Design review of the part built by this model. Coordinates are the model's own, in mm. A direction names the side the tool comes from. Coordinates: 2 decimals unless noted, no trailing zeros. Loops run counter-clockwise (first coordinate to the right, second up) from the corner with the lowest first, then second, coordinate; pieces in that order, holes last. Notation, with made-up numbers: M 11.5,82.5 L 67.5,82.5 A11 cw 67.5,92.5 Z; hole C 4.5,-39.5 d3. An arc over 180 degrees is marked long. Answer as a JSON object with one key per item and string values. Group by question number.
1. Consider section A-A (x = 0). State the section outline as (y, z) points.
2. Insertion check: pin 1 (6 mm diameter, centred on y = 3.5, z = 20, fed in from +X); pin 2 (3.5 mm diameter, centred on x = 0, y = 0, fed in from +Z); pin 3 (1.5 mm diameter, centred on x = 5.5, z = 9, fed in from +Y). Each pin has a flat end and moves straight along its axis. Give the tip position at first contact, or say it passes through.
3. Consider section B-B (y = 0). State the section outline as (x, z) points.
4. Consider section D-D (z = 14.5). State the section outline as (x, y) points.
5. To check wall thickness, follow probe 1 along Y at (x, z) = (0, 29.75); probe 2 along Y at (x, z) = (0, 5.25); probe 3 along X at (y, z) = (-10.75, 14.5). State the ranges of each line that lie inside material, in increasing order.
6. Draft analysis for pull direction X (two halves, no side actions). For faces 4 (the flat face through (0, -3, 40)), 5 (the cylindrical face through (5.77, -11.09, 19.72)), 6 (the flat face through (0, 0, 25)), state which applies: +X half, -X half, draft (parallel to the pull), parting line (faces both ways), or undercut.
7. Machinability: for faces 1 (the flat face through (3, -3, 0)), 2 (the flat face through (0, 0, 10)), 3 (the cylindrical face through (0, -2, 33)), which of the approach directions +Z, -Z, +X, -X, +Y, -Y give a long, thin tool a straight path to every point of the face, cutting with its end or side? Answer none if there is none.
8. Consider section C-C (z = 6.5). State the section outline as (x, y) points.
from build123d import *

# Parameters (mm, degrees)
F0_R     = 12.5
F1_DEPTH = 40
F2_R     = 2
F3_DEPTH = 15
F4_R     = 3
F5_DEPTH = 10
F6_R     = 2.5
F7_DEPTH = 12.5


with BuildPart() as f1:
    # F0 (on Top) → F1 (new body)
    with BuildSketch(Plane.XY):
        Circle(F0_R)
    extrude(amount=F1_DEPTH)

    # F2 (on face) → F3 (cut)
    with BuildSketch(Plane.XY.offset(40)):
        Circle(F2_R)
    extrude(amount=-F3_DEPTH, mode=Mode.SUBTRACT)

    # F4 (on face) → F5 (cut)
    with BuildSketch(Plane(origin=(0, 0, 0), x_dir=(1, 0, 0), z_dir=(0, 0, -1))):
        Circle(F4_R)
    extrude(amount=-F5_DEPTH, mode=Mode.SUBTRACT)

    # F6 (on Front) → F7 (cut, symmetric)
    with BuildSketch(Plane.XZ):
        with Locations((0, 15)):
            Circle(F6_R)
    extrude(amount=F7_DEPTH, both=True, mode=Mode.SUBTRACT)


solid = f1.part
Findings below:
{
 "1": {"outline": "M -12.5,0 L -3,0 L -3,10 L 3,10 L 3,0 L 12.5,0 L 12.5,12.5 L -12.5,12.5 Z; M -12.5,17.5 L 12.5,17.5 L 12.5,40 L 2,40 L 2,25 L -2,25 L -2,40 L -12.5,40 Z"},
 "2": {"pin 1": "stops at x = 12.49", "pin 2": "stops at z = 25", "pin 3": "stops at y = 11.56"},
 "3": {"outline": "M -12.5,0 L -3,0 L -3,10 L 3,10 L 3,0 L 12.5,0 L 12.5,40 L 2,40 L 2,25 L -2,25 L -2,40 L -12.5,40 Z; hole C 0,15 d5"},
 "4": {"outline": "M -2.45,-12.26 L -2.45,12.26 A12.5 ccw Z; M 2.45,-12.26 A12.5 ccw 2.45,12.26 Z"},
 "5": {"probe 1": "y = -12.5 to -2, 2 to 12.5", "probe 2": "y = -12.5 to -3, 3 to 12.5", "probe 3": "x = -6.38 to -2.45, 2.45 to 6.38"},
 "6": {"face 4": "draft", "face 5": "parting line", "face 6": "undercut"},
 "7": {"face 1": "-Z, +X, -X, +Y, -Y", "face 2": "-Z", "face 3": "+Z"},
 "8": {"outline": "C 0,0 d25; hole C 0,0 d6"}
}
